Design review of the part shown in the three views and the two pictorial views. Dimensions are in mm from the part's minimum x, y and z. Round coordinates to 2 decimals unless told otherwise and drop trailing zeros. Order: outer loops, then holes, each group sorted by start corner. A loop starts at its lowest first (then second) coordinate and runs counter-clockwise, first axis right, second up.
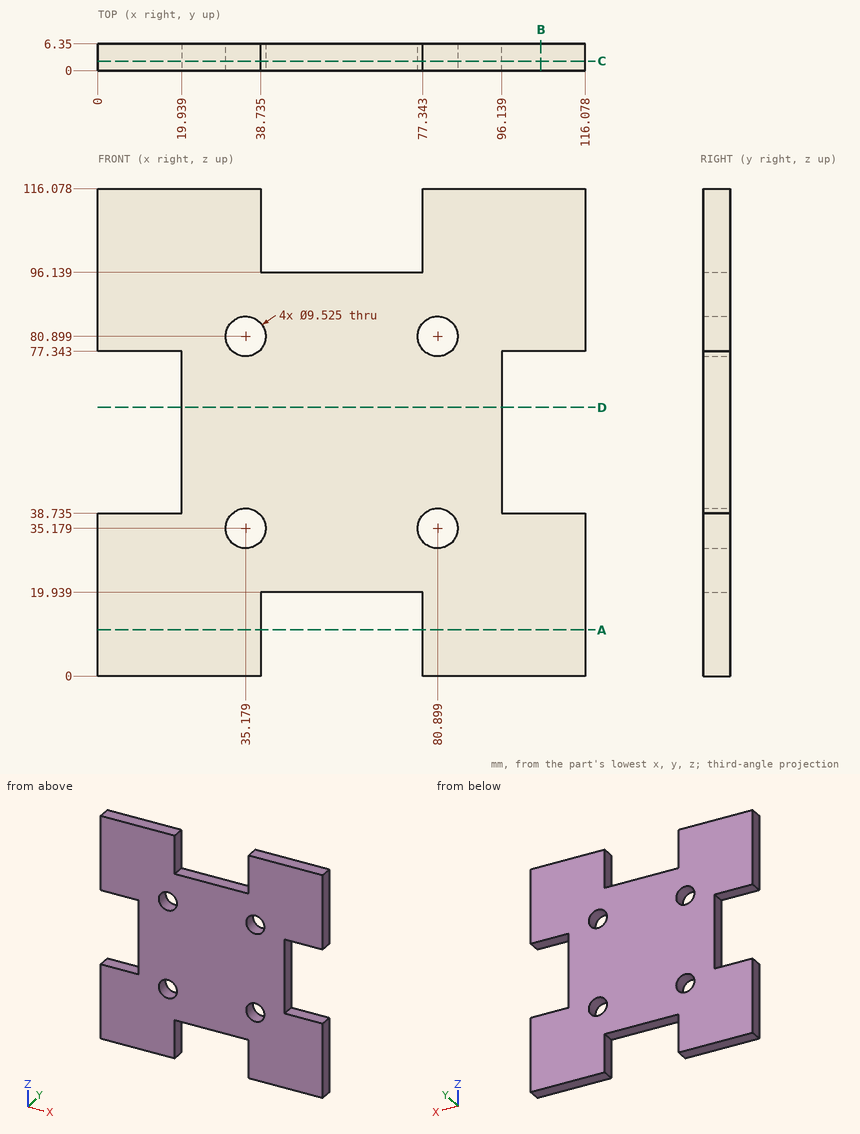
(1) Add section C-C on y = 2.25. Give the boundary of the cut face in (x, z) (1 decimal).
(2) Add section B-B on x = 105.5. Give the boundary of the cut face in (y, z) (3 decimals).
(3) Clearance check with flat-ended pins moving along their axes: P1, Ø15, axis at x = 80.899, z = 80.899, coming from the +Y side; P2, Ø3, axis at y = 4, z = 66.5, coming from the +X side; P3, Ø3, axis at y = 4, z = 58.5, coming from the -X side. State where each tip first meets the part, or that it passes through.
(4) Add section D-D on z = 64. Give the boundary of the cut face in (x, y).
(5) Add section A-A on z = 11. Give the boundary of the cut face in (x, y) (3 decimals).
(6) Wall thickness on L1, parallel to Z at x = 18, y = 2.25 (3 decimals); L2, parallel to X at y = 4.75, z = 81.5; L3, parallel to X at y = 5, z = 76.5: over which ranges is each line inside the solid? List them lowest first.
Here are the results:
1. outline: (0, 0) - (38.7, 0) - (38.7, 19.9) - (77.3, 19.9) - (77.3, 0) - (116.1, 0) - (116.1, 38.7) - (96.1, 38.7) - (96.1, 77.3) - (116.1, 77.3) - (116.1, 116.1) - (77.3, 116.1) - (77.3, 96.1) - (38.7, 96.1) - (38.7, 116.1) - (0, 116.1) - (0, 77.3) - (19.9, 77.3) - (19.9, 38.7) - (0, 38.7) - close; hole circle Ø9.5 at (35.2, 35.2); hole circle Ø9.5 at (35.2, 80.9); hole circle Ø9.5 at (80.9, 35.2); hole circle Ø9.5 at (80.9, 80.9)
2. outline: (0, 0) - (6.35, 0) - (6.35, 38.735) - (0, 38.735) - close; (0, 77.343) - (6.35, 77.343) - (6.35, 116.078) - (0, 116.078) - close
3. P1: stops at y = 6.35
3. P2: stops at x = 96.14
3. P3: stops at x = 19.94
4. outline: (19.94, 0) - (96.14, 0) - (96.14, 6.35) - (19.94, 6.35) - close
5. outline: (0, 0) - (38.735, 0) - (38.735, 6.35) - (0, 6.35) - close; (77.343, 0) - (116.078, 0) - (116.078, 6.35) - (77.343, 6.35) - close
6. L1: z = 0 to 38.735, 77.343 to 116.078
6. L2: x = 0 to 30.45, 39.9 to 76.17, 85.62 to 116.08
6. L3: x = 19.94 to 33.35, 37 to 79.07, 82.72 to 96.14
